The listing builds one solid part. Answer for the finished solid, in the listing's coordinates (mm). A direction names the side the tool comes from. Give positions to 0.01 mm unless a question says otherwise; leave off trailing zeros. Loops run counter-clockwise (first coordinate to the right, second up) from the corner with the lowest first, then second, coordinate; pieces in that order, holes last. Notation, with made-up numbers: (7.5, 66.25) - (30.5, 66.25) arc R15 ccw to (30.5, 70.25) - close; hole circle Ø2 at (45.5, 54). An arc over 180 degrees is marked (long way). One line per item, written item: value. Start each with the question number.
from build123d import *

# Parameters (mm, degrees)
F0_W     = 96
F0_H     = 24
F1_DEPTH = 2
F2_W     = 36
F2_H     = 2
F3_DEPTH = 36
F2_W_2   = 92
F2_W_3   = 2
F2_H_2   = 20
F2_W_4   = 28
F4_DEPTH = 16
F5_SIZE  = 19.99999
F6_DEPTH = 2


# Not quite as in the source:
# - a fillet or chamfer is up to 0.001 mm smaller than in the source, because OpenCascade refuses the exact size


with BuildPart() as f1:
    # F0 (on Top) → F1 (new body)
    with BuildSketch(Plane.XY):
        with Locations((48, 12)):
            Rectangle(F0_W, F0_H)
    extrude(amount=F1_DEPTH)

    # F2 (on face) → F3 (join)
    with BuildSketch(Plane.XY.offset(2)):
        with Locations((48, 1)):
            Rectangle(F2_W, F2_H)
    extrude(amount=F3_DEPTH)

    # F2 (on face) → F4 (join)
    with BuildSketch(Plane.XY.offset(2)):
        with Locations((48, 23)):
            Rectangle(F2_W_2, F2_H)
        with Locations((95, 23)):
            Rectangle(F2_W_3, F2_H)
        with Locations((48, 1)):
            Rectangle(F2_W, F2_H)
        with Locations((95, 12)):
            Rectangle(F2_W_3, F2_H_2)
        with Locations((95, 1)):
            Rectangle(F2_W_3, F2_H)
        Polygon((2, 22), (2, 24), (0, 24), (0, 2), (2, 2), align=None)
        with Locations((1, 1)):
            Rectangle(F2_W_3, F2_H)
        with Locations((16, 1)):
            Rectangle(F2_W_4, F2_H)
        with Locations((80, 1)):
            Rectangle(F2_W_4, F2_H)
    extrude(amount=F4_DEPTH)

    # F5 (size 20 in the source; OpenCascade refuses exactly that, so slightly less here)
    f5_edges = [f1.edges().sort_by_distance(p)[0] for p in [
        (30, 1, 18),
        (66, 1, 18),
    ]]
    chamfer(f5_edges, length=F5_SIZE)

    # F0 (on Top) → F6 (join, through all)
    with BuildSketch(Plane.XY):
        Polygon((96, 0), (0, 0), (28, -12), (68, -12), align=None)
    extrude(amount=F6_DEPTH)


solid = f1.part
1. A cutting plane is placed at C-C (x = 46.5). Determine the outline of the cut face in (y, z), plus the area to 3 significant figures.
2. Determine the mould class of faces 1 (the flat face through (14, -6, 1)), 2 (the flat face through (47, 22, 10)), 3 (the flat face through (76, 1, 28)) for opening direction Y: released by +Y, released by -Y, zero draft, split by the parting line, or undercut.
3. A cutting plane is placed at A-A (y = 20). Determine the outline of the cut face in (x, z), plus the area to 3 significant figures.
4. For faces 4 (the flat face through (49, 2, 16)), 5 (the flat face through (49, 24, 9)), 6 (the flat face through (47, -5, 2)), determine the directions among +Z, -Z, +X, -X, +Y, -Y from which every point of the face is accessible in a straight line to the end or side of a thin tool.
5. Find the intervals of material crossed by L1, parallel to X at y = 10.5, z = 14.5; L2, parallel to Y at x = 65, z = 17; L3, parallel to Y at x = 69.5, z = 32.5, in increasing order. Write a range as [from, to].
6. A cutting plane is placed at B-B (z = 13.5). Determine the outline of the cut face in (x, y), plus the area to 3 significant figures.
7. A cutting plane is placed at D-D (x = 71.5). Determine the outline of the cut face in (y, z), plus the area to 3 significant figures.
8. Flat-ended cylindrical pins translate along their axes: pin 1 (3.5 mm diameter, centred on x = 41, y = -7, fed in from +Z); pin 2 (6 mm diameter, centred on x = 31, z = 20.5, fed in from -Y). Find the tip coordinate at first contact, or state that the pin passes through.
Results below:
1. outline: (-12, 0) - (24, 0) - (24, 18) - (22, 18) - (22, 2) - (2, 2) - (2, 38) - (0, 38) - (0, 2) - (-12, 2) - close
1. area: 176 mm^2
2. face 1: released by -Y
2. face 2: undercut
2. face 3: zero draft
3. outline: (0, 0) - (96, 0) - (96, 18) - (94, 18) - (94, 2) - (2, 2) - (2, 18) - (0, 18) - close
3. area: 256 mm^2
4. face 4: +Z
4. face 5: +Z, -Z, +X, -X, +Y
4. face 6: +Z, +X, -X, -Y
5. L1: x = [0, 2], [94, 96]
5. L2: y = [0, 2], [22, 24]
5. L3: y = [0, 2]
6. outline: (0, 0) - (96, 0) - (96, 24) - (0, 24) - close; hole (2, 2) - (94, 2) - (94, 22) - (2, 22) - close
6. area: 464 mm^2
7. outline: (-10.5, 0) - (24, 0) - (24, 18) - (22, 18) - (22, 2) - (2, 2) - (2, 32.5) - (0, 32.5) - (0, 2) - (-10.5, 2) - close
7. area: 162 mm^2
8. pin 1: stops at z = 2
8. pin 2: stops at y = 0
